Read the model definition and answer for the solid it produces. Units are mm, in the model's axes. Face numbers are marked on the shaded views. A direction names the side the tool comes from. Round coordinates to 2 decimals unless told otherwise and drop trailing zeros. Order: outer loops, then holes, each group sorted by start corner. A loop starts at its lowest first (then second) coordinate and runs counter-clockwise, first axis right, second up.
from build123d import *

# Parameters (mm, degrees)
BOSS_EXTRUDE1_DEPTH      = 10
SKETCH2_R                = 1.75
CUT_EXTRUDE1_DEPTH       = 10
SKETCH3_R                = 1.25
SKETCH3_R_2              = 1.8
CUT_EXTRUDE2_DEPTH       = 40.143965052
SKETCH4_W                = 13.022509218
SKETCH4_H                = 4.5
CUT_EXTRUDE3_DEPTH       = 40.143965052
BOSS_EXTRUDE2_DEPTH      = 10
BOSS_EXTRUDE2_DEPTH_BACK = 10
SKETCH5_W                = 12.5
SKETCH5_H                = 1.5
LOFT2_DEPTH              = 2.5


# Read off the part's stored shape, not the designer's step: Loft2
with BuildPart() as part:
    # Sketch1 → Boss-Extrude1 (new body)
    with BuildSketch(Plane.XY):
        Polygon((0, 0), (0, 36.5), (12.5, 36.5), (12.5, 34), (2.5, 34), (2.5, 0), align=None)
    extrude(amount=BOSS_EXTRUDE1_DEPTH)

    # Sketch2 → Cut-Extrude1 (cut)
    with BuildSketch(Plane.XZ.offset(-34)):
        with Locations((7.5, 5)):
            Circle(SKETCH2_R)
    extrude(amount=-CUT_EXTRUDE1_DEPTH, mode=Mode.SUBTRACT)

    # Sketch3 → Cut-Extrude2 (cut, through all)
    with BuildSketch(Plane(origin=(2.5, 0, 0), x_dir=(0, 0, -1), z_dir=(1, 0, 0))):
        with Locations(Location((-3.25, 7.15, 0), (0, 0, 90))):
            Circle(SKETCH3_R)
        with Locations(Location((-3.25, 16.85, 0), (0, 0, 270))):
            Circle(SKETCH3_R)
        with Locations(Location((-5, 29, 0), (0, 0, 90))):
            Circle(SKETCH3_R_2)
    extrude(amount=-CUT_EXTRUDE2_DEPTH, mode=Mode.SUBTRACT)

    # Sketch4 → Cut-Extrude3 (cut, through all)
    with BuildSketch(Plane(origin=(2.5, 0, 0), x_dir=(0, 0, -1), z_dir=(1, 0, 0))):
        with Locations((-6.511254609, 2.25)):
            Rectangle(SKETCH4_W, SKETCH4_H)
    extrude(amount=-CUT_EXTRUDE3_DEPTH, mode=Mode.SUBTRACT)

    # Sketch5 → Boss-Extrude2 (add, two sides: drawn at the far end of the back side and taken through both)
    with BuildSketch(Plane.XY.offset(10).offset(-BOSS_EXTRUDE2_DEPTH_BACK)):
        with Locations((6.25, 23.15)):
            Rectangle(SKETCH5_W, SKETCH5_H)
    extrude(amount=BOSS_EXTRUDE2_DEPTH + BOSS_EXTRUDE2_DEPTH_BACK)

    # Loft2 outline → Loft2 (add)
    with BuildSketch(Plane.YZ):
        Polygon((22.4, 10), (22.4, 20), (4.5, 10), align=None)
    extrude(amount=LOFT2_DEPTH)


solid = part.part
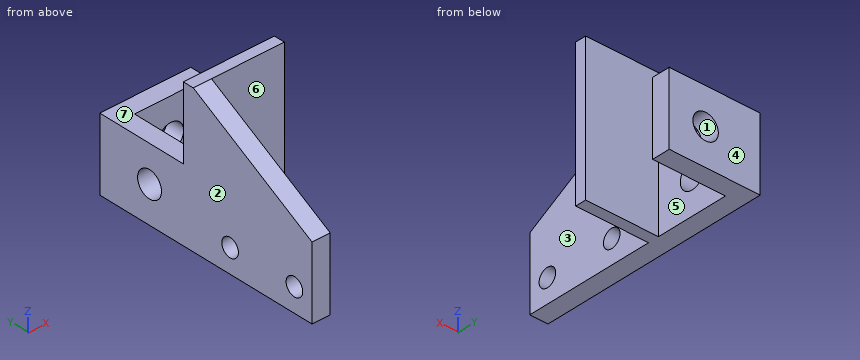
Q1. A cutting plane is placed at D-D, the plane x = 11. Give the vertices of the cut face in (y, z).
Outcome:
outline: (22.4, 0) - (23.9, 0) - (23.9, 20) - (22.4, 20) - close; (34, 0) - (36.5, 0) - (36.5, 10) - (34, 10) - close
Q2. For a pull along X with two mould halves and no side action, classify the marked faces 1, 2, 3 and 4 as released by +X, released by -X, zero draft, split by the parting line, or undercut.
Outcome:
face 1: undercut
face 2: released by -X
face 3: released by +X
face 4: zero draft
Q3. Flat-ended cylindrical pins translate along their axes: pin 1 (9 mm diameter, centred on y = 15, z = 10, fed in from +X); pin 2 (3 mm diameter, centred on x = 5.5, y = 11.5, fed in from +Z); pin 3 (5 mm diameter, centred on x = 6, z = 17.5, fed in from -Y); pin 4 (6 mm diameter, centred on x = 6.5, z = 5, fed in from +Y). Find the tip coordinate at first contact, or state that the pin passes through.
Outcome:
pin 1: stops at x = 2.5
pin 2: passes through
pin 3: stops at y = 22.4
pin 4: stops at y = 36.5
Q4. A cutting plane is placed at C-C, the plane y = 29. Give the vertices of the cut face in (x, z), plus the area to 3 significant figures.
Outcome:
outline: (0, 0) - (2.5, 0) - (2.5, 3.2) - (0, 3.2) - close; (0, 6.8) - (2.5, 6.8) - (2.5, 10) - (0, 10) - close
area: 16.0 mm2
Q5. A cutting plane is placed at A-A, the plane z = 5. Give the vertices of the cut face in (x, y).
Outcome:
outline: (0, 4.5) - (2.5, 4.5) - (2.5, 22.4) - (12.5, 22.4) - (12.5, 23.9) - (2.5, 23.9) - (2.5, 27.2) - (0, 27.2) - close; (0, 30.8) - (2.5, 30.8) - (2.5, 34) - (5.75, 34) - (5.75, 36.5) - (0, 36.5) - close; (9.25, 34) - (12.5, 34) - (12.5, 36.5) - (9.25, 36.5) - close
Q6. Straight lines are drawn through the part: probe 1 along Z at (x, y) = (1.1, 29); probe 2 along Y at (x, z) = (6.25, 13); probe 3 along Z at (x, y) = (2.25, 16). For each, find the intervals that lie inside material, in ascending order.
Outcome:
probe 1: z = 0 to 3.2, 6.8 to 10
probe 2: y = 22.4 to 23.9
probe 3: z = 0 to 2.33, 4.17 to 16.42
Q7. A cutting plane is placed at B-B, the plane x = 7.5. Give the vertices of the cut face in (y, z), plus the area to 4 significant figures.
Outcome:
outline: (22.4, 0) - (23.9, 0) - (23.9, 20) - (22.4, 20) - close; (34, 0) - (36.5, 0) - (36.5, 3.25) - (34, 3.25) - close; (34, 6.75) - (36.5, 6.75) - (36.5, 10) - (34, 10) - close
area: 46.25 mm2
Q8. For the marked faces 5, 6 and 7, determine the directions among +Z, -Z, +X, -X, +Y, -Y from which every point of the face is accessible in a straight line to the end or side of a thin tool.
Outcome:
face 5: +Z, -Z, +X
face 6: +Z, -Z, +X, -Y
face 7: +Z, +X, -X, +Y
